The listing builds one solid part. Answer for the finished solid, in the listing's coordinates (mm). Face numbers are marked on the shaded views. A direction names the side the tool comes from. Round coordinates to 2 decimals unless told otherwise and drop trailing zeros. Loops run counter-clockwise (first coordinate to the right, second up) from the corner with the lowest first, then second, coordinate; pieces in that order, holes last. Notation, with made-up numbers: M -7.5,50.5 L 3.5,50.5 A32 cw 3.5,82.5 Z; hole C 17,-36 d7. An arc over 180 degrees is marked long. Put each result on its own line as item: value. Start each with the question number.
(1) Section B-B, the plane y = 58 is taken. Determine the outline of the cut face in (x, z), then the cut area to 4 significant figures.
(2) Determine the mould class of the marked faces 3, 4 and 5 for opening direction Y: released by +Y, released by -Y, zero draft, split by the parting line, or undercut.
(3) Section C-C, the plane x = 18 is taken. Determine the outline of the cut face in (y, z), then the cut area to 3 significant figures.
(4) Straight lines are drawn through the part: line 1 (X direction, y = 70.55, z = 19); line 2 (Y direction, x = 60.5, z = 4.5); line 3 (Y direction, x = 53, z = 1.3). For each, find the intervals that lie inside material, in ascending order.
(5) Section A-A, the plane z = 13.75 is taken. Determine the outline of the cut face in (x, y), then the cut area to 3 significant figures.
(6) Flat-ended cylindrical pins translate along their axes: P1, Ø2, axis at x = 26.5, y = 33.5, coming from the +Z side; P2, Ø2.5, axis at y = 71, z = 13.5, coming from the +X side. Find the tip coordinate at first contact, or state that the pin passes through.
(7) Which of the six approach directions +Z, -Z, +X, -X, +Y, -Y give full straight-line access (tool end or side, diameter ignored) to the marked faces 1 and 2?
(8) Section D-D, the plane y = 21.35 is taken. Determine the outline of the cut face in (x, z), then the cut area to 3 significant figures.
```python
from build123d import *

# Parameters (mm, degrees)
SKETCH_4_R          = 1.65
EXTRUDE_1_DEPTH     = 3
SKETCH_5_W          = 63
SKETCH_5_H          = 3
EXTRUDE_2_DEPTH     = 20
SKETCH_6_R          = 1.65
SKETCH_6_W          = 10
SKETCH_6_H          = 20
CUT_EXTRUDE_1_DEPTH = 100
FILLET_2_R          = 2


with BuildPart() as part:
    # 草图4 → 凸台-拉伸1 (new body)
    with BuildSketch(Plane.XY):
        with BuildLine():
            Line((75, 69), (75, 72))
            Line((75, 72), (12, 72))
            Line((12, 72), (12, 36))
            Line((12, 36), (12, 0))
            Line((12, 0), (75, 0))
            Line((75, 0), (75, 3))
            ThreePointArc((75, 3), (92.66106403, 36), (75, 69))
        make_face()
        with Locations((22, 14)):
            Circle(SKETCH_4_R, mode=Mode.SUBTRACT)
        with Locations((30, 14)):
            Circle(SKETCH_4_R, mode=Mode.SUBTRACT)
        with Locations((22, 21.35)):
            Circle(SKETCH_4_R, mode=Mode.SUBTRACT)
        with Locations((22, 29.35)):
            Circle(SKETCH_4_R, mode=Mode.SUBTRACT)
        with Locations((53, 14)):
            Circle(SKETCH_4_R, mode=Mode.SUBTRACT)
        with Locations((65, 14)):
            Circle(SKETCH_4_R, mode=Mode.SUBTRACT)
        with Locations((73, 14)):
            Circle(SKETCH_4_R, mode=Mode.SUBTRACT)
        with BuildLine():
            ThreePointArc((26.65, 36), (25, 34.35), (23.35, 36))
            ThreePointArc((23.35, 36), (25, 37.65), (26.65, 36))
        make_face(mode=Mode.SUBTRACT)
        with Locations((22, 42.65)):
            Circle(SKETCH_4_R, mode=Mode.SUBTRACT)
        with Locations((22, 50.65)):
            Circle(SKETCH_4_R, mode=Mode.SUBTRACT)
        with Locations((22, 58)):
            Circle(SKETCH_4_R, mode=Mode.SUBTRACT)
        with Locations((30, 58)):
            Circle(SKETCH_4_R, mode=Mode.SUBTRACT)
        with Locations((81, 36)):
            Circle(SKETCH_4_R, mode=Mode.SUBTRACT)
        with Locations((53, 58)):
            Circle(SKETCH_4_R, mode=Mode.SUBTRACT)
        with Locations((65, 58)):
            Circle(SKETCH_4_R, mode=Mode.SUBTRACT)
        with Locations((73, 58)):
            Circle(SKETCH_4_R, mode=Mode.SUBTRACT)
        with Locations((53, 43)):
            Circle(SKETCH_4_R, mode=Mode.SUBTRACT)
        with Locations((53, 29)):
            Circle(SKETCH_4_R, mode=Mode.SUBTRACT)
        with Locations((46, 36)):
            Circle(SKETCH_4_R, mode=Mode.SUBTRACT)
        with Locations((53, 36)):
            Circle(SKETCH_4_R, mode=Mode.SUBTRACT)
        with Locations((60, 36)):
            Circle(SKETCH_4_R, mode=Mode.SUBTRACT)
    extrude(amount=EXTRUDE_1_DEPTH)

    # 草图5 → 凸台-拉伸2 (add)
    with BuildSketch(Plane.XY.offset(3)):
        with Locations((43.5, 70.5)):
            Rectangle(SKETCH_5_W, SKETCH_5_H)
        with Locations((43.5, 1.5)):
            Rectangle(SKETCH_5_W, SKETCH_5_H)
    extrude(amount=EXTRUDE_2_DEPTH)

    # 草图6 → 切除-拉伸1 (cut)
    with BuildSketch(Plane(origin=(0, 72, 0), x_dir=(1, 0, 0), z_dir=(0, 1, 0))):
        with Locations(Location((18, -11, 0), (0, 0, 270))):
            Circle(SKETCH_6_R)
        with Locations(Location((18, -19, 0), (0, 0, 270))):
            Circle(SKETCH_6_R)
        with Locations(Location((26, -19, 0), (0, 0, 270))):
            Circle(SKETCH_6_R)
        with Locations(Location((26, -11, 0), (0, 0, 270))):
            Circle(SKETCH_6_R)
        with Locations(Location((61, -11, 0), (0, 0, 270))):
            Circle(SKETCH_6_R)
        with Locations(Location((61, -19, 0), (0, 0, 270))):
            Circle(SKETCH_6_R)
        with Locations(Location((69, -19, 0), (0, 0, 270))):
            Circle(SKETCH_6_R)
        with Locations(Location((69, -11, 0), (0, 0, 270))):
            Circle(SKETCH_6_R)
        with Locations((38.5, -13)):
            Rectangle(SKETCH_6_W, SKETCH_6_H)
        with Locations((48.5, -13)):
            Rectangle(SKETCH_6_W, SKETCH_6_H)
    extrude(amount=-CUT_EXTRUDE_1_DEPTH, mode=Mode.SUBTRACT)

    # 圆角2
    fillet_2_edges = [part.edges().sort_by_distance(p)[0] for p in [
        (12, 70.5, 23),
        (75, 70.5, 23),
        (12, 1.5, 23),
        (75, 1.5, 23),
        (33.5, 1.5, 23),
        (53.5, 1.5, 23),
        (53.5, 70.5, 23),
        (33.5, 70.5, 23),
    ]]
    fillet(fillet_2_edges, radius=FILLET_2_R)


solid = part.part
```
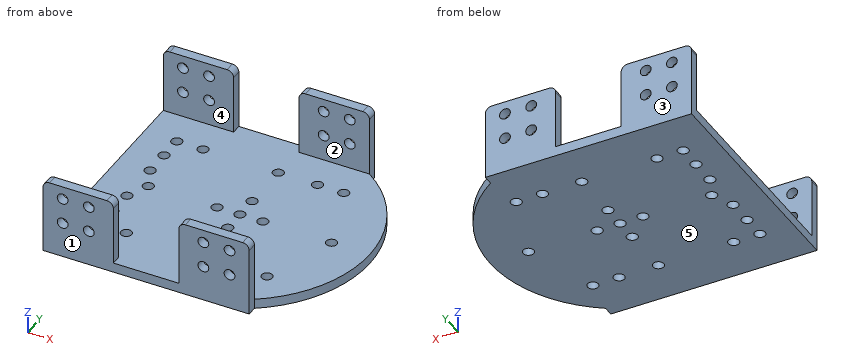
Recorded:
1. outline: M 12,0 L 20.35,0 L 20.35,3 L 12,3 Z; M 23.65,0 L 28.35,0 L 28.35,3 L 23.65,3 Z; M 31.65,0 L 51.35,0 L 51.35,3 L 31.65,3 Z; M 54.65,0 L 63.35,0 L 63.35,3 L 54.65,3 Z; M 66.65,0 L 71.35,0 L 71.35,3 L 66.65,3 Z; M 74.65,0 L 86,0 L 86,3 L 74.65,3 Z
1. area: 172.5 mm²
2. face 3: released by +Y
2. face 4: undercut
2. face 5: zero draft
3. outline: M 0,0 L 72,0 L 72,9.35 L 69,9.35 L 69,3 L 3,3 L 3,9.35 L 0,9.35 Z; M 0,12.65 L 3,12.65 L 3,17.35 L 0,17.35 Z; M 0,20.65 L 3,20.65 L 3,23 L 0,23 Z; M 69,12.65 L 72,12.65 L 72,17.35 L 69,17.35 Z; M 69,20.65 L 72,20.65 L 72,23 L 69,23 Z
3. area: 296 mm²
4. line 1: x = 12 to 16.35, 19.65 to 24.35, 27.65 to 33.5, 53.5 to 59.35, 62.65 to 67.35, 70.65 to 75
4. line 2: y = 0 to 3, 69 to 72
4. line 3: y = 0 to 12.35, 15.65 to 27.35, 30.65 to 34.35, 37.65 to 41.35, 44.65 to 56.35, 59.65 to 72
5. outline: M 12,0 L 33.5,0 L 33.5,3 L 12,3 Z; M 12,69 L 33.5,69 L 33.5,72 L 12,72 Z; M 53.5,0 L 75,0 L 75,3 L 53.5,3 Z; M 53.5,69 L 75,69 L 75,72 L 53.5,72 Z
5. area: 258 mm²
6. P1: stops at z = 3
6. P2: stops at x = 75
7. face 1: +Z, -Z, +X, -X, -Y
7. face 2: +Z, +X, -X
8. outline: M 12,0 L 20.35,0 L 20.35,3 L 12,3 Z; M 23.65,0 L 89.86,0 L 89.86,3 L 23.65,3 Z
8. area: 224 mm²
